The drawing under review shows one solid part. Ordinate dimensions are in mm from its lowest x, y, z. A direction names the side the tool comes from. Coordinates: 2 decimals unless noted, no trailing zeros. Write each loop counter-clockwise with the first axis right and the second up, starting at its lowest first coordinate (ties: lowest second). Pieces come first, ordered by that corner, then holes. Notation, with made-up numbers: (87.25, 69) - (131.25, 69) arc R23 cw to (131.25, 105) - close; hole circle Ø10 at (85, 32.25). An arc over 180 degrees is marked (long way). Use a Markdown table: item, result.
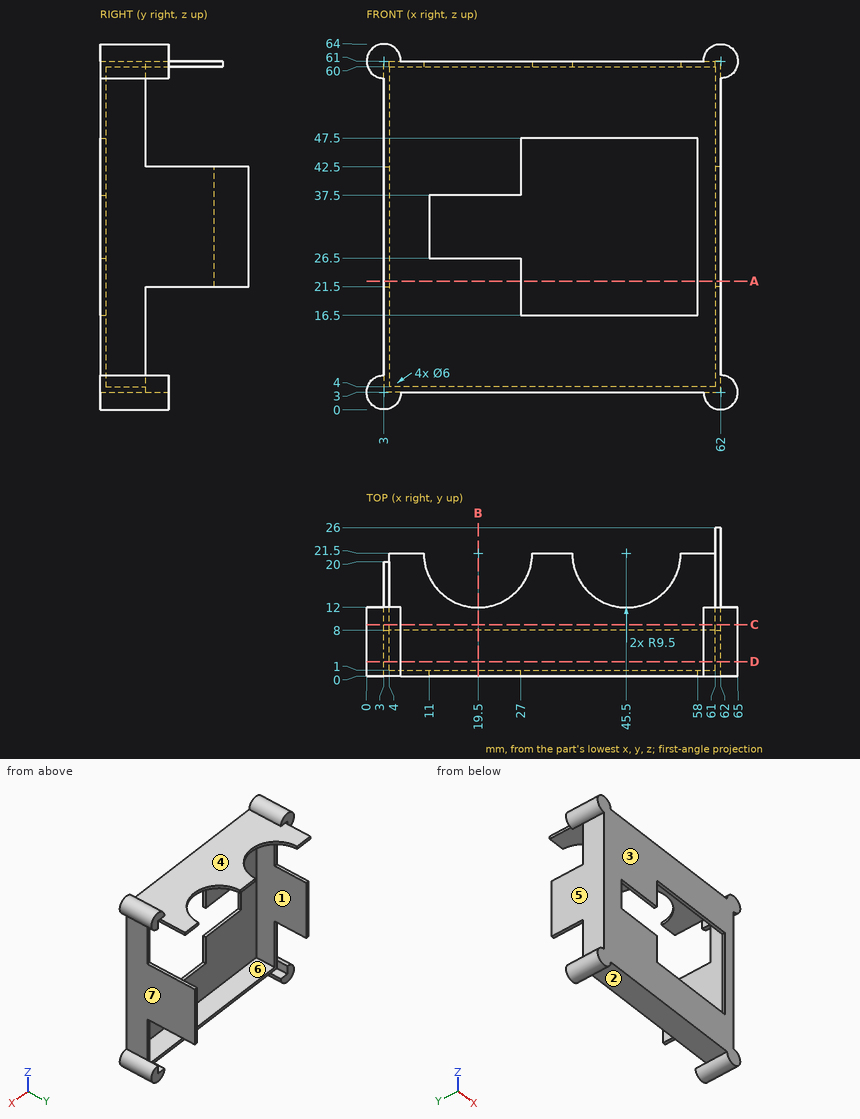
(1) Take a section at C-C on y = 9. Write out the cut boundary in (x, z).
Determined:
| item | result |
|---|---|
| outline | (3, 3) - (3, 6) arc R3 ccw (long way) to (6, 3) - close; (3, 21.5) - (4, 21.5) - (4, 42.5) - (3, 42.5) - close; (3, 58) - (3, 61) - (4, 61) - (4, 60) - (61, 60) - (61, 61) - (62, 61) - (62, 58) arc R3 ccw (long way) to (59, 61) - (6, 61) arc R3 ccw (long way) to start; (59, 3) arc R3 ccw (long way) to (62, 6) - (62, 3) - close; (61, 21.5) - (62, 21.5) - (62, 42.5) - (61, 42.5) - close |
(2) Take a section at D-D on y = 2.5. Write out the cut boundary in (x, z), and give its area (3 significant figures).
Determined:
| item | result |
|---|---|
| outline | (3, 6) arc R3 ccw (long way) to (6, 3) - (59, 3) arc R3 ccw (long way) to (62, 6) - (62, 58) arc R3 ccw (long way) to (59, 61) - (6, 61) arc R3 ccw (long way) to (3, 58) - close; hole (4, 4) - (61, 4) - (61, 60) - (4, 60) - close |
| area | 315 mm2 |
(3) Take a section at A-A on z = 22.5. Write out the cut boundary in (x, y).
Determined:
| item | result |
|---|---|
| outline | (3, 0) - (27, 0) - (27, 1) - (4, 1) - (4, 20) - (3, 20) - close; (58, 0) - (62, 0) - (62, 26) - (61, 26) - (61, 1) - (58, 1) - close |
(4) Machinability: for the marked faces 5, 6 and 7, which of the approach directions +Z, -Z, +X, -X, +Y, -Y give a long, thin tool a straight path to every point of the face, cutting with its end or side? Answer none if there is none.
Determined:
| item | result |
|---|---|
| face 5 | -X, +Y, -Y |
| face 6 | +Y |
| face 7 | +X, +Y, -Y |
(5) For pin 1 (1.5 mm diameter, centred on x = 22.5, y = 10.5, fed in from +Z); pin 2 (10 mm diameter, centred on y = 3.5, z = 45, fed in from +X); pin 3 (1.1 mm diameter, centred on x = 3.5, z = 35, fed in from +Y); pin 4 (5 mm diameter, centred on x = 29.5, z = 28, fed in from +Y), all flat-tipped, find the tip position at first contact; note any pin that passes through.
Determined:
| item | result |
|---|---|
| pin 1 | z = 61 |
| pin 2 | x = 62 |
| pin 3 | y = 20 |
| pin 4 | through |
(6) Take a section at B-B on x = 19.5. Write out the cut boundary in (y, z), and give its area (3 significant figures).
Determined:
| item | result |
|---|---|
| outline | (0, 3) - (8, 3) - (8, 4) - (1, 4) - (1, 26.5) - (0, 26.5) - close; (0, 37.5) - (1, 37.5) - (1, 60) - (12, 60) - (12, 61) - (0, 61) - close |
| area | 65.0 mm2 |
(7) For L1, parallel to Z at x = 8.5, y = 7.5; L2, parallel to X at y = 1.75, z = 56; L3, parallel to Y at x = 60.5, z = 19, list the stretches that pass through material, from the lowest coordinate up. Write a range as from..to.
Determined:
| item | result |
|---|---|
| L1 | 3..4, 60..61 |
| L2 | 3..4, 61..62 |
| L3 | 0..1 |
(8) Draft analysis for pull direction Z (two halves, no side actions). For the marked faces 1, 2, 3 and 4, state which applies: +Z half, -Z half, draft (parallel to the pull), parting line (faces both ways), or undercut.
Determined:
| item | result |
|---|---|
| face 1 | undercut |
| face 2 | -Z half |
| face 3 | draft |
| face 4 | +Z half |
